Work out the finished part from the listing and answer in its coordinate system (mm). Coordinates: 2 decimals unless noted, no trailing zeros. Order: outer loops, then holes, each group sorted by start corner. A loop starts at its lowest first (then second) coordinate and runs counter-clockwise, first axis right, second up. Notation, with made-up numbers: M 69,-11.75 L 118,-11.75 A15 ccw 118,11.25 Z; hole C -7.75,12 d2. An arc over 180 degrees is marked long. Answer in a Markdown table with one row per item. Add a question column.
Item 1: Consider line 1 (X direction, y = 28, z = 3.5); line 2 (Y direction, x = 14, z = 12); line 3 (Y direction, x = 46.5, z = 6.75). Determine where each line is inside the solid, lowest interval first. Write a range as from..to.
Item 2: The part is cut by section A-A (y = 21.5). Write down the section's boundary in (x, z), then the cut area to 3 significant figures.
Item 3: The part is cut by section B-B (y = 16). Write down the section's boundary in (x, z), then the cut area to 3 significant figures.
Item 4: The part is cut by section C-C (z = 9.75). Write down the section's boundary in (x, y).
Item 5: The part is cut by section D-D (x = 63.5). Write down the section's boundary in (y, z), then the cut area to 3 significant figures.
Item 6: Flat-ended cylindrical pins translate along their axes: pin 1 Ø8 at (x, z) = (25, 6) entering from +Y; pin 2 Ø5.5 at (x, z) = (32.5, 2) entering from +Y; pin 3 Ø8 at (x, z) = (30.5, 16) entering from -Y. Find the tip coordinate at first contact, or state that the pin passes through.
from build123d import *

# Parameters (mm, degrees)
F1_DEPTH = 5
F3_W     = 70
F3_H     = 15
F3_W_2   = 60
F3_H_2   = 5


with BuildPart() as f1:
    # F0 (on Top) → F1 (new body)
    with BuildSketch(Plane.XY):
        Polygon((0, 50), (0, 0), (70, 0), (70, 50), (55, 50), (55, 15), (15, 15), (15, 50), align=None)
    extrude(amount=F1_DEPTH)

    # F4: sweep along a path in F2
    with BuildLine(Plane(origin=(0, 0, 0), x_dir=(0, -1, 0), z_dir=(-1, 0, 0))) as f4_path:
        Line((0, 5), (-5.1303021499, 19.0953893118))
    # F3 (on face) → F4 (sweep)
    with BuildSketch(Plane.XY.offset(5)):
        with Locations((35, 7.5)):
            Rectangle(F3_W, F3_H)
        with Locations((35, 7.5)):
            Rectangle(F3_W_2, F3_H_2, mode=Mode.SUBTRACT)
    sweep(path=f4_path.line)


solid = f1.part
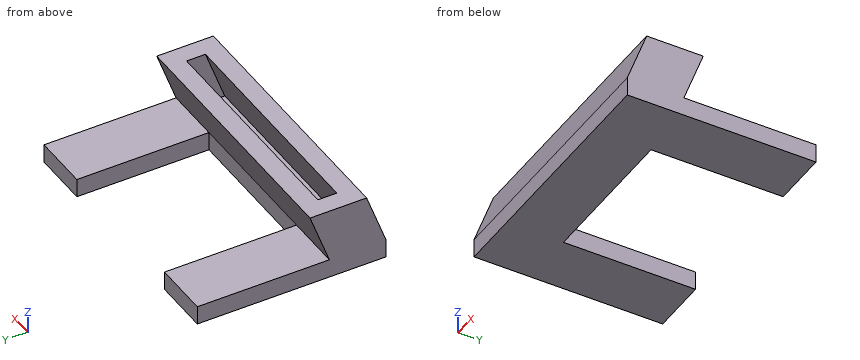
Reply:
| question | item | result |
|---|---|---|
| 1 | line 1 | x = 0..15, 55..70 |
| 1 | line 2 | y = 2.55..7.55, 12.55..17.55 |
| 1 | line 3 | y = 0.64..5.64, 10.64..15.64 |
| 2 | outline | M 0,0 L 15,0 L 15,5 L 0,5 Z; M 55,0 L 70,0 L 70,5 L 55,5 Z |
| 2 | area | 150 mm2 |
| 3 | outline | M 0,0 L 15,0 L 15,5 L 0,5 Z; M 0,7.75 L 70,7.75 L 70,19.1 L 0,19.1 Z; M 55,0 L 70,0 L 70,5 L 55,5 Z |
| 3 | area | 944 mm2 |
| 4 | outline | M 0,1.73 L 70,1.73 L 70,16.73 L 0,16.73 Z; hole M 5,6.73 L 65,6.73 L 65,11.73 L 5,11.73 Z |
| 5 | outline | M 0,0 L 50,0 L 50,5 L 15,5 L 20.13,19.1 L 15.13,19.1 L 10,5 L 5,5 L 10.13,19.1 L 5.13,19.1 L 0,5 Z |
| 5 | area | 391 mm2 |
| 6 | pin 1 | stops at y = 16.82 |
| 6 | pin 2 | stops at y = 15 |
| 6 | pin 3 | stops at y = 2.55 |
